from build123d import *

# Parameters (mm, degrees)
CYLINDER1283_R     = 1
CYLINDER1283_DEPTH = 20
CYLINDER1280_R     = 1
CYLINDER1280_DEPTH = 20
CYLINDER1279_R     = 2.6
CYLINDER1279_DEPTH = 12
CYLINDER1293_R     = 7
CYLINDER1293_DEPTH = 9


with BuildPart() as obj1:
    # Cylinder1283 → Cylinder1283 (new body)
    with BuildSketch(Plane(origin=(-3.5, -3.5, 0), x_dir=(1, 0, 0), z_dir=(0, 0, 1))):
        Circle(CYLINDER1283_R)
    extrude(amount=CYLINDER1283_DEPTH)


with BuildPart() as compound693:
    # Cylinder1280 → Cylinder1280 (new body)
    with BuildSketch(Plane(origin=(3.5, 3.5, 0), x_dir=(1, 0, 0), z_dir=(0, 0, 1))):
        Circle(CYLINDER1280_R)
    extrude(amount=CYLINDER1280_DEPTH)

    # Compound693: union obj1
    add(obj1.part)


with BuildPart() as obj2:
    # Cylinder1279 → Cylinder1279 (new body)
    with BuildSketch(Plane.XY.offset(13)):
        Circle(CYLINDER1279_R)
    extrude(amount=CYLINDER1279_DEPTH)


with BuildPart() as cut484:
    # Cylinder1293 → Cylinder1293 (new body)
    with BuildSketch(Plane.XY.offset(13)):
        Circle(CYLINDER1293_R)
    extrude(amount=CYLINDER1293_DEPTH)

    # Cut490: cut obj2
    add(obj2.part, mode=Mode.SUBTRACT)


with BuildPart() as cut484_1:
    # Cut490 placement: moved
    add(cut484.part.moved(Location((0, 0, -2))))

    # Cut484: cut Compound693
    add(compound693.part, mode=Mode.SUBTRACT)


solid = cut484_1.part
Geometry check sheet. Reference: the model listing, model coordinates, mm. Give positions to 0.01 mm unless a question says otherwise; leave off trailing zeros. Order: outer loops, then holes, each group sorted by start corner. A loop starts at its lowest first (then second) coordinate and runs counter-clockwise, first axis right, second up.
1. Depth check by flat-ended pin: pin 1 (1 mm diameter, centred on y = 2.5, z = 18.5, fed in from -X); pin 2 (1.6 mm diameter, centred on x = 3.5, y = 3.5, fed in from -Z); pin 3 (5 mm diameter, centred on y = -1.5, z = 18, fed in from -X); pin 4 (3 mm diameter, centred on y = -2.5, z = 15, fed in from +X). Enter the tip coordinate at first touch or a pass-through.
Completed:
pin 1: stops at x = -6.71
pin 2: passes through
pin 3: stops at x = -7
pin 4: stops at x = 6.93
2. Scan lines: line 1 (Y direction, x = -3.5, z = 17); line 2 (Y direction, x = 0, z = 14); line 3 (X direction, y = 3.5, z = 17.25). Record each from-to range of solid material in increasing order.
Completed:
line 1: y = -6.06 to -4.5, -2.5 to 6.06
line 2: y = -7 to -2.6, 2.6 to 7
line 3: x = -6.06 to 2.5, 4.5 to 6.06
3. Sectioned sample at C-C (z = 18.5). Record the boundary of the cut face in (x, y), then the cut area to 3 significant figures.
Completed:
outline: circle Ø14 at (0, 0); hole circle Ø2 at (-3.5, -3.5); hole circle Ø5.2 at (0, 0); hole circle Ø2 at (3.5, 3.5)
area: 126 mm2
4. Sectioned sample at A-A (x = 0). Record the boundary of the cut face in (y, z).
Completed:
outline: (-7, 11) - (-2.6, 11) - (-2.6, 20) - (-7, 20) - close; (2.6, 11) - (7, 11) - (7, 20) - (2.6, 20) - close
5. Draft check along Y on faces 1 (the face through (6.466, -2.681, 15.437)), 2 (the face through (0, -3, 11)), 3 (the face through (-0.338, 2.578, 15.437)), 4 (the face through (-4.5, -3.5, 15.4)). Enter one of: pulls with the +Y half, pulls with the -Y half, needs draft (parallel to the pull), parting line crosses it, or undercut.
Completed:
face 1: parting line crosses it
face 2: needs draft
face 3: undercut
face 4: undercut
6. Sectioned sample at D-D (y = 5.5). Record the boundary of the cut face in (x, z).
Completed:
outline: (-4.33, 11) - (4.33, 11) - (4.33, 20) - (-4.33, 20) - close
